Answer from the drawing. Dimensions are ordinates in mm from the lowest x, y and z of the part. A direction names the side the tool comes from. Coordinates: 2 decimals unless noted, no trailing zeros. Loops run counter-clockwise (first coordinate to the right, second up) from the corner with the lowest first, then second, coordinate; pieces in that order, holes last.
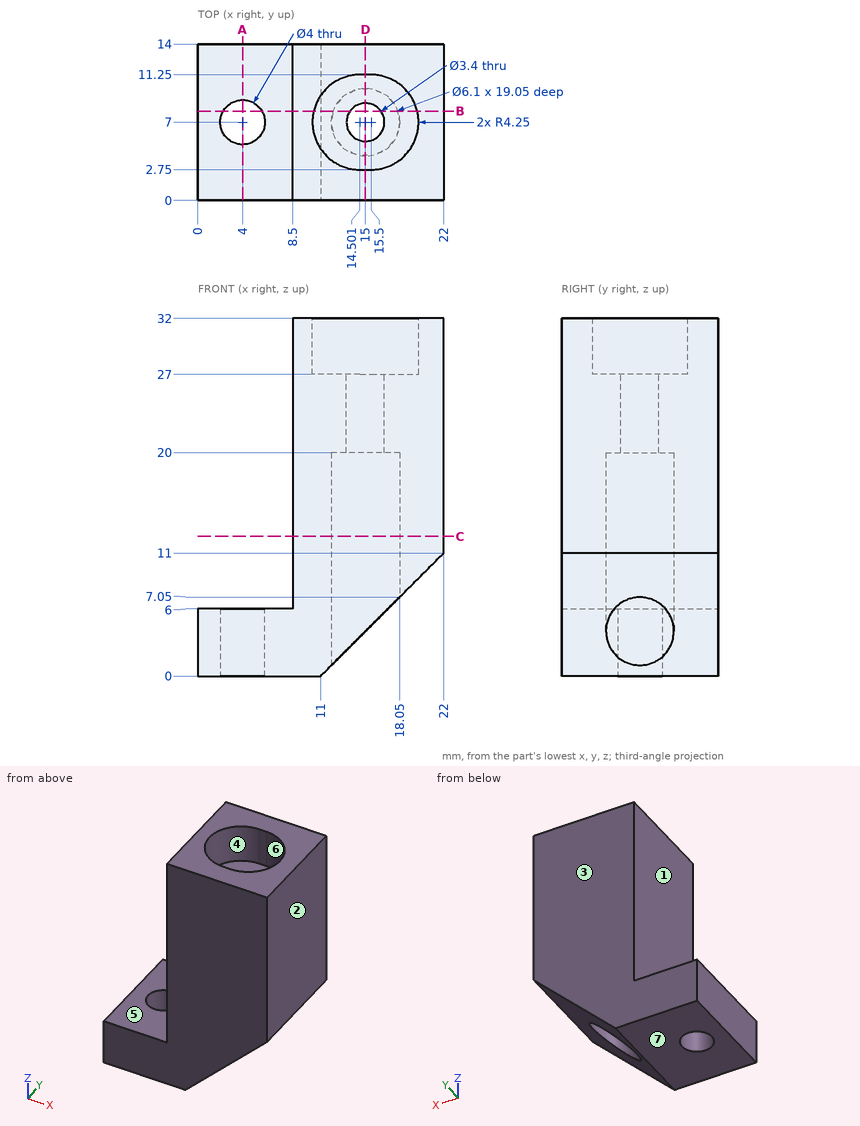
Item 1: A cutting plane is placed at A-A on x = 4. Determine the outline of the cut face in (y, z).
Numbers:
outline: (0, 0) - (5, 0) - (5, 6) - (0, 6) - close; (9, 0) - (14, 0) - (14, 6) - (9, 6) - close
Item 2: Given pin 1 (8 mm diameter, centred on x = 15.5, y = 8, fed in from -Z); pin 2 (1.8 mm diameter, centred on x = 16, y = 8, fed in from -Z); pin 3 (7 mm diameter, centred on x = 3, y = 10.5, fed in from +Z); pin 4 (2.5 mm diameter, centred on x = 4, y = 7, fed in from -Z), each flat-ended and moving along its own axis, determine where each tip first touches the part or whether it passes through.
Numbers:
pin 1: stops at z = 0.5
pin 2: stops at z = 20
pin 3: stops at z = 6
pin 4: passes through
Item 3: Determine the mould class of the marked faces 1, 2, 3 and 4 for opening direction X: released by +X, released by -X, zero draft, split by the parting line, or undercut.
Numbers:
face 1: released by -X
face 2: released by +X
face 3: zero draft
face 4: undercut
Item 4: Which of the six approach directions +Z, -Z, +X, -X, +Y, -Y give full straight-line access (tool end or side, diameter ignored) to the marked faces 5, 6 and 7?
Numbers:
face 5: +Z, -X, +Y, -Y
face 6: +Z
face 7: -Z, +X, -X, +Y, -Y
Item 5: A cutting plane is placed at B-B on y = 8. Determine the outline of the cut face in (x, z) (1 decimal).
Numbers:
outline: (0, 0) - (2.3, 0) - (2.3, 6) - (0, 6) - close; (5.7, 0) - (11, 0) - (12.1, 1.1) - (12.1, 20) - (13.6, 20) - (13.6, 27) - (10.4, 27) - (10.4, 32) - (8.5, 32) - (8.5, 6) - (5.7, 6) - close; (16.4, 20) - (17.9, 20) - (17.9, 6.9) - (22, 11) - (22, 32) - (19.6, 32) - (19.6, 27) - (16.4, 27) - close
Item 6: Find the intervals of material crossed by line 1 along Y through (x, z) = (15, 25.25); line 2 along X through (y, z) = (7, 13); line 3 along X through (y, z) = (7, 24), in increasing order.
Numbers:
line 1: y = 0 to 5.3, 8.7 to 14
line 2: x = 8.5 to 11.95, 18.05 to 22
line 3: x = 8.5 to 13.3, 16.7 to 22
Item 7: A cutting plane is placed at D-D on x = 15. Determine the outline of the cut face in (y, z), then the cut area to 3 significant figures.
Numbers:
outline: (0, 4) - (3.95, 4) - (3.95, 20) - (5.3, 20) - (5.3, 27) - (2.75, 27) - (2.75, 32) - (0, 32) - close; (8.7, 20) - (10.05, 20) - (10.05, 4) - (14, 4) - (14, 32) - (11.25, 32) - (11.25, 27) - (8.7, 27) - close
area: 228 mm2
Item 8: A cutting plane is placed at C-C on z = 12.5. Determine the outline of the cut face in (x, y).
Numbers:
outline: (8.5, 0) - (22, 0) - (22, 14) - (8.5, 14) - close; hole circle Ø6.1 at (15, 7)
